Verification items for the finished model (mm, model axes). A direction names the side the tool comes from. Give positions to 0.01 mm unless a question says otherwise; leave off trailing zeros. Order: outer loops, then holes, each group sorted by start corner. A loop starts at its lowest first (then second) coordinate and runs counter-clockwise, first axis right, second up. Notation, with made-up numbers: (42.5, 61) -> (58.5, 61) arc R30 cw to (58.5, 84) -> close; hole circle Ø4 at (50.25, -6). An arc over 180 degrees is marked (long way). One line per question, with ' | ' between items. Start each with the question number.
Q1. Access from +Z, -Z, +X, -X, +Y, -Y to the whole of each face (thin tool, end or side, straight path). Record for faces 1 (the cylindrical face through (-1.172, 8.923, 39.746)), 2 (the cylindrical face through (-1.172, 8.923, 11.106)), 3 (the flat face through (-7, -6, 31.5)).
Q2. Section check A-A on y = 0. Record the cut outline in (x, z), plus the area to 4 significant figures.
Q3. Material ranges on probe 1 along Z at (x, y) = (-8.75, -6); probe 2 along Y at (x, z) = (-0.25, 37); probe 3 along X at (y, z) = (-1, 10.5), recorded low to high. Write a range as [from, to].
Q4. Section check C-C on z = 31. Record the cut outline in (x, y), plus the area to 3 significant figures.
Q5. Go/stop test with flat-tipped pins: pin 1 (12 mm diameter, centred on y = 8.5, z = 31.5, fed in from -X) (3 decimals); pin 2 (11.5 mm diameter, centred on x = -2.5, y = 0, fed in from -Z); pin 3 (10 mm diameter, centred on x = -6.5, z = 27.5, fed in from +Y); pin 4 (8 mm diameter, centred on y = -4.5, z = 11, fed in from +X). Record where each tip stops, or that it passes through.
from build123d import *

# Parameters (mm, degrees)
SKETCH1_R           = 9
BOSS_EXTRUDE1_DEPTH = 40
BOSS_EXTRUDE5_START = -0.5
SKETCH4_R           = 11.5
BOSS_EXTRUDE5_DEPTH = 8
BOSS_EXTRUDE6_START = 2
SKETCH5_R           = 11.5
BOSS_EXTRUDE6_DEPTH = 8
SKETCH6_R           = 9
SKETCH6_R_2         = 8.75
CUT_EXTRUDE1_DEPTH  = 1


with BuildPart() as part:
    # Sketch1 → Boss-Extrude1 (new body)
    with BuildSketch(Plane.XY):
        Circle(SKETCH1_R)
    extrude(amount=BOSS_EXTRUDE1_DEPTH)

    # Sketch4 → Boss-Extrude5 (add)
    with BuildSketch(Plane.XY.offset(40).offset(BOSS_EXTRUDE5_START)):
        Circle(SKETCH4_R)
    extrude(amount=-BOSS_EXTRUDE5_DEPTH)

    # Sketch5 → Boss-Extrude6 (add)
    with BuildSketch(Plane(origin=(0, 0, 31.5), x_dir=(-1, 0, 0), z_dir=(0, 0, -1)).offset(BOSS_EXTRUDE6_START)):
        with Locations(Location((0, 0, 0), (0, 0, 180))):
            Circle(SKETCH5_R)
    extrude(amount=BOSS_EXTRUDE6_DEPTH)

    # Sketch6 → Cut-Extrude1 (cut)
    with BuildSketch(Plane(origin=(0, 0, 0), x_dir=(-1, 0, 0), z_dir=(0, 0, -1))):
        Circle(SKETCH6_R)
        Circle(SKETCH6_R_2, mode=Mode.SUBTRACT)
    extrude(amount=-CUT_EXTRUDE1_DEPTH, mode=Mode.SUBTRACT)


solid = part.part
Filled in:
1) face 1: +Z | face 2: -Z | face 3: none
2) outline: (-11.5, 21.5) -> (-9, 21.5) -> (-9, 1) -> (-8.75, 1) -> (-8.75, 0) -> (8.75, 0) -> (8.75, 1) -> (9, 1) -> (9, 21.5) -> (11.5, 21.5) -> (11.5, 29.5) -> (9, 29.5) -> (9, 31.5) -> (11.5, 31.5) -> (11.5, 39.5) -> (9, 39.5) -> (9, 40) -> (-9, 40) -> (-9, 39.5) -> (-11.5, 39.5) -> (-11.5, 31.5) -> (-9, 31.5) -> (-9, 29.5) -> (-11.5, 29.5) -> close | area: 799.5 mm²
3) probe 1: [21.5, 29.5], [31.5, 39.5] | probe 2: [-11.5, 11.5] | probe 3: [-8.94, 8.94]
4) outline: circle Ø18 at (0, 0) | area: 254 mm²
5) pin 1: x = -11.225 | pin 2: z = 0 | pin 3: y = 11.4 | pin 4: x = 8.99
